Design review of the part shown in the three views and the two pictorial views. Dimensions are in mm from the part's minimum x, y and z. A direction names the side the tool comes from. Give positions to 0.01 mm unless a question says otherwise; leave off trailing zeros. Loops run counter-clockwise (first coordinate to the right, second up) from the corner with the lowest first, then second, coordinate; pieces in that order, holes last.
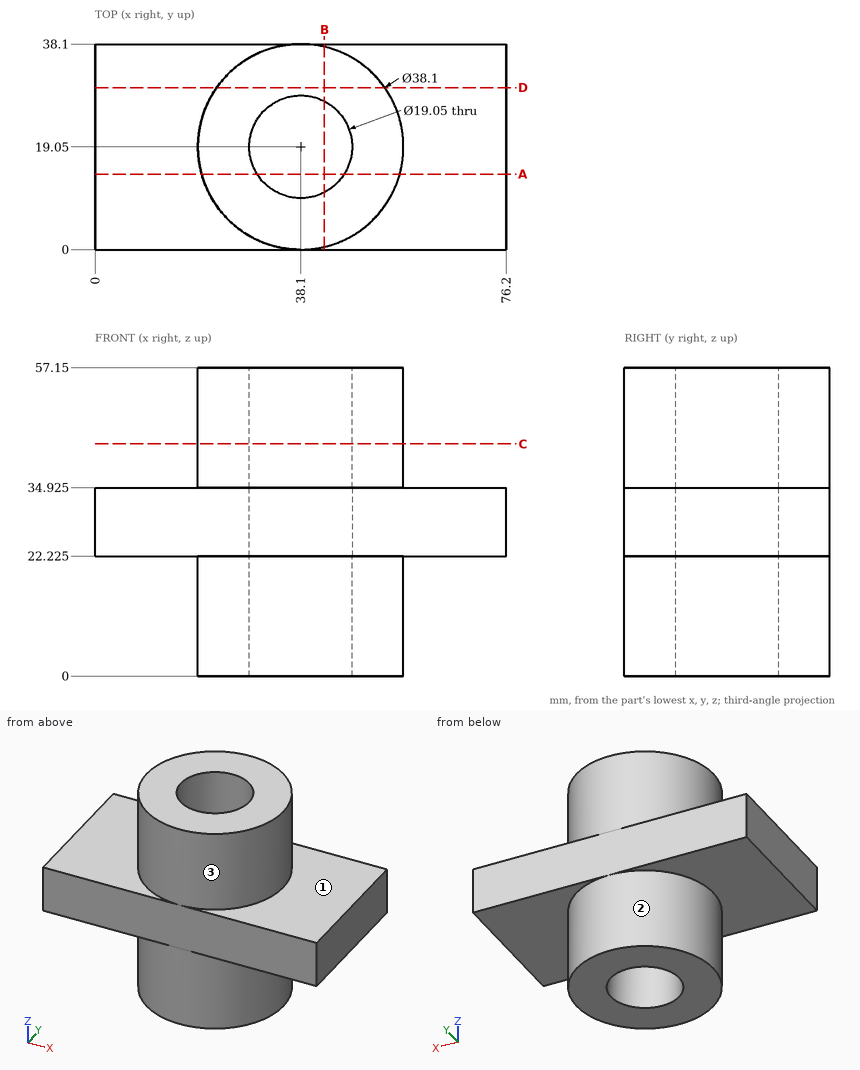
Q1. Take a section at D-D (y = 30). Give the boundary of the cut face in (x, z) (3 decimals), plus the area to 3 significant figures.
Results:
outline: (0, 22.225) - (22.512, 22.225) - (22.512, 0) - (53.688, 0) - (53.688, 22.225) - (76.2, 22.225) - (76.2, 34.925) - (53.688, 34.925) - (53.688, 57.15) - (22.512, 57.15) - (22.512, 34.925) - (0, 34.925) - close
area: 2,350 mm2
Q2. Take a section at A-A (y = 14). Give the boundary of the cut face in (x, z) (3 decimals).
Results:
outline: (0, 22.225) - (19.732, 22.225) - (19.732, 0) - (30.024, 0) - (30.024, 57.15) - (19.732, 57.15) - (19.732, 34.925) - (0, 34.925) - close; (46.176, 0) - (56.468, 0) - (56.468, 22.225) - (76.2, 22.225) - (76.2, 34.925) - (56.468, 34.925) - (56.468, 57.15) - (46.176, 57.15) - close
Q3. Wall thickness on line 1 (X direction, y = 19, z = 44); line 2 (Y direction, x = 38.1, z = 9) (3 decimals); line 3 (Y direction, x = 33.5, z = 8): over which ranges is each line inside the solid? List them lowest first.
Results:
line 1: x = 19.05 to 28.58, 47.62 to 57.15
line 2: y = 0 to 9.525, 28.575 to 38.1
line 3: y = 0.56 to 10.71, 27.39 to 37.54
Q4. Take a section at B-B (x = 42.5). Give the boundary of the cut face in (y, z) (3 decimals), plus the area to 3 significant figures.
Results:
outline: (0, 22.225) - (0.515, 22.225) - (0.515, 0) - (10.602, 0) - (10.602, 57.15) - (0.515, 57.15) - (0.515, 34.925) - (0, 34.925) - close; (27.498, 0) - (37.585, 0) - (37.585, 22.225) - (38.1, 22.225) - (38.1, 34.925) - (37.585, 34.925) - (37.585, 57.15) - (27.498, 57.15) - close
area: 1,170 mm2
Q5. Insertion check: pin 1 (5 mm diameter, centred on x = 9.5, y = 16, fed in from +Z) (3 decimals); pin 2 (6 mm diameter, centred on x = 45.5, z = 42, fed in from -Y); pin 3 (2 mm diameter, centred on y = 20, z = 19.5, fed in from +X); pin 4 (17 mm diameter, centred on x = 38.1, y = 19.05, fed in from +Z). Each pin has a flat end and moves straight along its axis. Give the tip position at first contact, or say it passes through.
Results:
pin 1: stops at z = 34.925
pin 2: stops at y = 0.52
pin 3: stops at x = 57.15
pin 4: passes through
Q6. Take a section at C-C (z = 43). Give the boundary of the cut face in (x, y) (3 decimals).
Results:
outline: circle Ø38.1 at (38.1, 19.05); hole circle Ø19.05 at (38.1, 19.05)
Q7. Tool access review of the marked faces 1, 2 and 3: name each direction out of +Z, -Z, +X, -X, +Y, -Y from which nothing blocks a thin tool from reaching the whole face with its end or side.
Results:
face 1: +Z, +X
face 2: -Z
face 3: +Z
